```python
from build123d import *

# Parameters (mm, degrees)
SKETCH_R        = 12.5
SKETCH_R_2      = 4.5
SKETCH_R_3      = 1.6
PAD_DEPTH       = 10
SKETCH001_R     = 4
PAD001_DEPTH    = 28
CHAMFER_SIZE    = 2
CHAMFER001_SIZE = 1


with BuildPart() as part:
    # Sketch → Pad (new body)
    with BuildSketch(Plane.XY):
        Circle(SKETCH_R)
        Circle(SKETCH_R_2, mode=Mode.SUBTRACT)
        with Locations((-6.717514, 6.717514)):
            Circle(SKETCH_R_3, mode=Mode.SUBTRACT)
        with Locations((5.656854, 5.656854)):
            Circle(SKETCH_R_3, mode=Mode.SUBTRACT)
        with Locations((6.717514, -6.717514)):
            Circle(SKETCH_R_3, mode=Mode.SUBTRACT)
        with Locations((-5.656854, -5.656854)):
            Circle(SKETCH_R_3, mode=Mode.SUBTRACT)
    extrude(amount=PAD_DEPTH)

    # Sketch001 → Pad001 (join)
    with BuildSketch(Plane.YZ.offset(-8)):
        with Locations((0, 5)):
            Circle(SKETCH001_R)
    extrude(amount=-PAD001_DEPTH)

    # Chamfer
    chamfer_edges = [part.edges().sort_by_distance(p)[0] for p in [
        (-36, -4, 5),
    ]]
    chamfer(chamfer_edges, length=CHAMFER_SIZE)

    # Chamfer001
    chamfer001_edges = [part.edges().sort_by_distance(p)[0] for p in [
        (4.056854, 5.656854, 10),
        (5.117514, -6.717514, 10),
        (-7.256854, -5.656854, 10),
        (-8.317514, 6.717514, 10),
    ]]
    chamfer(chamfer001_edges, length=CHAMFER001_SIZE)


solid = part.part
```
Read the model definition and answer for the solid it produces. Units are mm, in the model's axes. A direction names the side the tool comes from. Give positions to 0.01 mm unless a question says otherwise; leave off trailing zeros. Loops run counter-clockwise (first coordinate to the right, second up) from the corner with the lowest first, then second, coordinate; pieces in that order, holes last.
Item 1: Find the intervals of material crossed by line 1 along Y through (x, z) = (0, 7.5); line 2 along X through (y, z) = (-7, 7.25); line 3 along X through (y, z) = (7, 4.5), in increasing order.
Item 2: The part is cut by section C-C (z = 8.25). Give the number of separate pieces and of enclosed holes in the cut face, and give its area (3 significant figures).
Item 3: The part is cut by section B-B (x = 0). Write down the section's boundary in (y, z).
Item 4: The part is cut by section A-A (y = 0). Write down the section's boundary in (x, z).
Item 5: The part is cut by section D-D (y = -10). Write down the section's boundary in (x, z).
Item 6: For faces 1 (the cylindrical face through (-22.766, -0.867, 1.095)), 2 (the flat face through (0, -5, 0)), determine the directions among +Z, -Z, +X, -X, +Y, -Y from which every point of the face is accessible in a straight line to the end or side of a thin tool.
Item 7: The mould has two halves that part along Y. Classify faces 3 (the flat face through (-36, 0, 5)), 4 (the cylindrical face through (-5.19, 7.2, 4.44)), 5 (the cylindrical face through (11.923, 3.755, 4.93)), 6 (the cylindrical face through (-0.59, 4.46, 4.93)): released by +Y, released by -Y, zero draft, split by the parting line, or undercut.
Item 8: Each of these flat-tipped pins is pushed along its axis until it touches: pin 1 Ø1 at (x, z) = (5, 1) entering from -Y; pin 2 Ø1 at (x, y) = (5, 7) entering from -Z; pin 3 Ø3.5 at (x, y) = (6.72, -6.72) entering from +Z; pin 4 Ø1 at (x, z) = (3.5, 3) entering from -Y. Where does it stop, or does it pass through?
Taken from the geometry:
1. line 1: y = -12.5 to -4.5, 4.5 to 12.5
1. line 2: x = -10.36 to -6.53, -4.79 to 5.14, 8.29 to 10.36
1. line 3: x = -10.36 to -8.29, -5.14 to 4.79, 6.53 to 10.36
2. separate pieces: 1
2. enclosed holes: 5
2. area: 498 mm2
3. outline: (-12.5, 0) - (-4.5, 0) - (-4.5, 10) - (-12.5, 10) - close; (4.5, 0) - (12.5, 0) - (12.5, 10) - (4.5, 10) - close
4. outline: (-36, 3) - (-34, 1) - (-12.5, 1) - (-12.5, 0) - (-4.5, 0) - (-4.5, 10) - (-12.5, 10) - (-12.5, 9) - (-34, 9) - (-36, 7) - close; (4.5, 0) - (12.5, 0) - (12.5, 10) - (4.5, 10) - close
5. outline: (-7.5, 0) - (7.5, 0) - (7.5, 10) - (-7.5, 10) - close
6. face 1: -X
6. face 2: -Z, +X, -X, +Y, -Y
7. face 3: zero draft
7. face 4: undercut
7. face 5: split by the parting line
7. face 6: undercut
8. pin 1: stops at y = -11.66
8. pin 2: stops at z = 0
8. pin 3: stops at z = 9.15
8. pin 4: stops at y = -12.13
